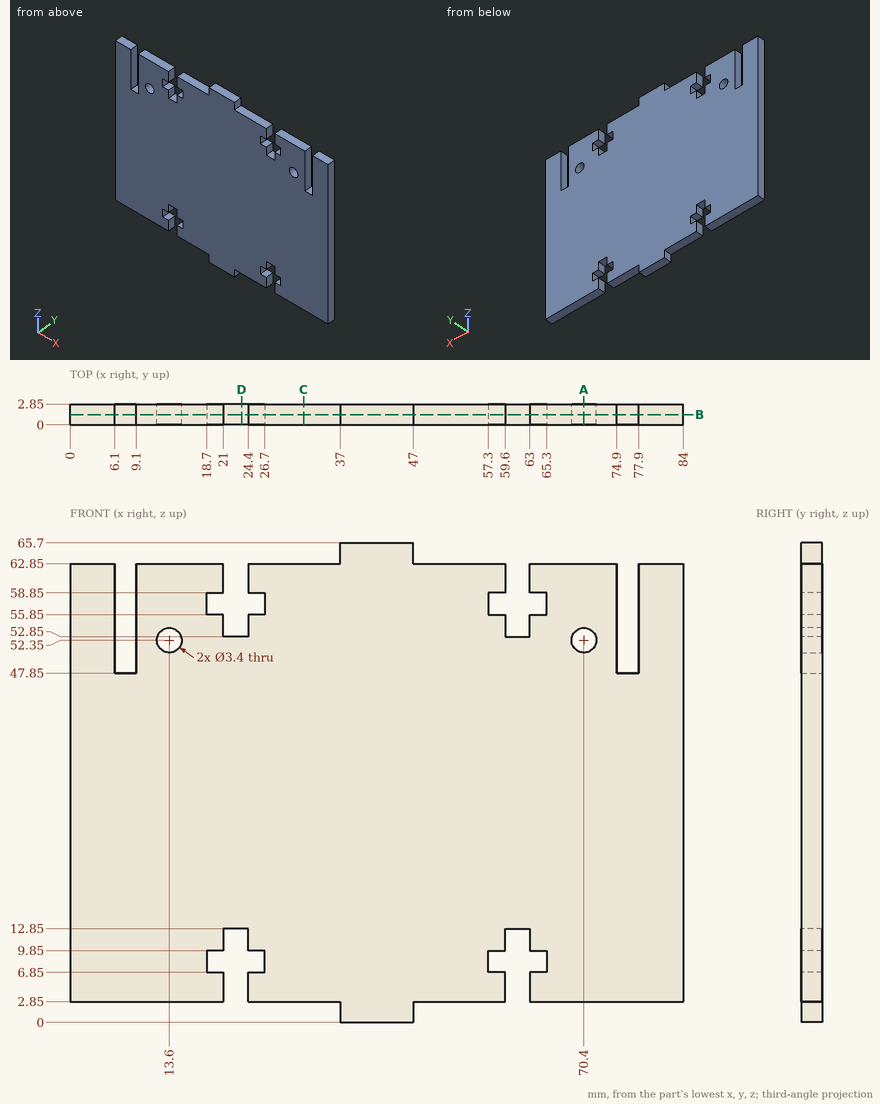
Geometry: see drawing. Coordinates: mm, zero at the bounding-box minimum. Give positions to 0.01 mm unless a question says otherwise; leave off trailing zeros. Loops run counter-clockwise (first coordinate to the right, second up) from the corner with the lowest first, then second, coordinate; pieces in that order, holes last. Notation, with made-up numbers: M 40.25,-28.75 L 78.25,-28.75 A11 ccw 78.25,-19.75 Z; hole C 14.5,-27.5 d5. An arc over 180 degrees is marked long. Use one line per item in the form item = value.
1. Section query A-A, the plane x = 70.4. Return the cut outline in (y, z).
Numbers:
outline = M 0,2.85 L 2.85,2.85 L 2.85,50.65 L 0,50.65 Z; M 0,54.05 L 2.85,54.05 L 2.85,62.85 L 0,62.85 Z
2. Section query D-D, the plane x = 23.5. Return the cut outline in (y, z), and give its area (3 significant figures).
Numbers:
outline = M 0,12.85 L 2.85,12.85 L 2.85,52.85 L 0,52.85 Z
area = 114 mm²
3. Section query B-B, the plane y = 1.4. Count the separate pieces of the cut face and the enclosed holes in it, and give its area (3 significant figures).
Numbers:
separate_pieces = 1
enclosed_holes = 2
area = 4,800 mm²
4. First-contact query: pin 1 (0.7 mm diameter, centred on x = 58, y = 2, fed in from +Z); pin 2 (0.9 mm diameter, centred on y = 2, z = 1, fed in from -X); pin 3 (1.4 mm diameter, centred on x = 77, y = 1.5, fed in from +Z). Flat tips, straight axial feed; report the tip coordinate or a pass-through.
Numbers:
pin_1 = 62.85
pin_2 = 37
pin_3 = 47.85
5. Section query C-C, the plane x = 32. Return the cut outline in (y, z), and give its area (3 significant figures).
Numbers:
outline = M 0,2.85 L 2.85,2.85 L 2.85,62.85 L 0,62.85 Z
area = 171 mm²
6. Line query: L1, parallel to X at y = 1.4, z = 52.35; L2, parallel to X at y = 0.75, z = 55.5; L3, parallel to X at y = 1, z = 10.5. Output: solid intervals per line, ascending.
Numbers:
L1 = 0 to 6.1, 9.1 to 11.9, 15.3 to 68.7, 72.1 to 74.9, 77.9 to 84
L2 = 0 to 6.1, 9.1 to 21, 24.4 to 59.6, 63 to 74.9, 77.9 to 84
L3 = 0 to 21, 24.4 to 59.6, 63 to 84
